Part model, mm, in its own coordinate system. A direction names the side the tool comes from. Round coordinates to 2 decimals unless told otherwise and drop trailing zeros. Write each loop counter-clockwise with the first axis right and the second up, starting at its lowest first coordinate (ties: lowest second). Pieces come first, ordered by that corner, then holes.
1) Which spindle directions (+Z, -Z, +X, -X, +Y, -Y) get a long thin tool onto all of the face, cutting with end or side? Do faces 1 (the flat face through (-51, 254, 22.309)), 2 (the flat face through (-51, 254, -0.691)), 3 (the flat face through (-32, 246, -1.691)). Say none if no direction does.
2) Flat gauge pins, fed straight in: pin 1 (0.8 mm diameter, centred on y = 266, z = 23, fed in from +X); pin 2 (2 mm diameter, centred on x = -52, y = 394, fed in from +Z); pin 3 (24 mm diameter, centred on x = -52.5, y = 151.5, fed in from -Z). Where does each tip first touch, or does it go through?
3) Saw through at A-A on y = 15. Write the cut outline in (x, z).
4) Pull direction Y, two halves, no side cores. Call faces 4 (the flat face through (-51, 500, 11)), 5 (the cylindrical face through (-46.285, 13.085, 10.97)), 6 (the flat face through (-75.904, 246, 11)): +Y half, -Y half, draft (parallel to the pull), parting line (faces both ways), or undercut.
5) Saw through at B-B on y = 301. Write the cut outline in (x, z), and give its area (3 significant figures).
6) Saw through at C-C on x = -41. Write the cut outline in (y, z).
7) Drill centre lines: L1, parallel to Y at x = -48, z = 21.75; L2, parallel to Z at x = -45, y = 388; L3, parallel to X at y = 153, z = 21.5. Where is each one in solid material? Low to high.
```python
from build123d import *

# Parameters (mm, degrees)
BOSS_EXTRUDE1_DEPTH              = 500
SKETCH3_W                        = 30
SKETCH3_H                        = 1
CUT_EXTRUDE1_DEPTH               = 500
M10X1_0_TAPPED_HOLE1_D           = 9
M10X1_0_TAPPED_HOLE1_DEPTH       = 51.26
M10X1_0_TAPPED_HOLE1_CBORE_D     = 10
M10X1_0_TAPPED_HOLE1_CBORE_DEPTH = 45.4
M10X1_0_TAPPED_HOLE1_TIP         = 2.703872786


with BuildPart() as part:
    # Sketch1 → Boss-Extrude1 (new body)
    with BuildSketch(Plane(origin=(0, 0, 0), x_dir=(1, 0, 0), z_dir=(0, 1, 0))):
        with BuildLine():
            Line((-73.903884132, 1.690933219), (-27.903884132, 1.690933219))
            ThreePointArc((-27.903884132, 1.690933219), (-26.48967057, 1.105146782), (-25.903884132, -0.309066781))
            Line((-25.903884132, -0.309066781), (-25.903884132, -21.309066781))
            ThreePointArc((-25.903884132, -21.309066781), (-26.48967057, -22.723280343), (-27.903884132, -23.309066781))
            Line((-27.903884132, -23.309066781), (-73.903884132, -23.309066781))
            ThreePointArc((-73.903884132, -23.309066781), (-75.318097695, -22.723280343), (-75.903884132, -21.309066781))
            Line((-75.903884132, -21.309066781), (-75.903884132, -0.309066781))
            ThreePointArc((-75.903884132, -0.309066781), (-75.318097695, 1.105146782), (-73.903884132, 1.690933219))
        make_face()
    extrude(amount=BOSS_EXTRUDE1_DEPTH)

    # Sketch3 → Cut-Extrude1 (cut)
    with BuildSketch(Plane(origin=(0, 500, 0), x_dir=(1, 0, 0), z_dir=(0, 1, 0))):
        with Locations((-50.903884132, 1.190933219)):
            Rectangle(SKETCH3_W, SKETCH3_H)
        with Locations((-50.903884132, -22.809066781)):
            Rectangle(SKETCH3_W, SKETCH3_H)
    extrude(amount=-CUT_EXTRUDE1_DEPTH, mode=Mode.SUBTRACT)

    # M10x1.0 Tapped Hole1
    with Locations(Plane(origin=(-50.903884132, 485, 22.309066781), x_dir=(1, 0, 0), z_dir=(0, 0, 1))):
        with Locations((0, 0), (0, -470)):
            CounterBoreHole(M10X1_0_TAPPED_HOLE1_D / 2, M10X1_0_TAPPED_HOLE1_CBORE_D / 2, M10X1_0_TAPPED_HOLE1_CBORE_DEPTH, depth=M10X1_0_TAPPED_HOLE1_DEPTH)
            with Locations((0, 0, -(M10X1_0_TAPPED_HOLE1_DEPTH + M10X1_0_TAPPED_HOLE1_TIP / 2))):  # 118° drill point
                Cone(0, M10X1_0_TAPPED_HOLE1_D / 2, M10X1_0_TAPPED_HOLE1_TIP, mode=Mode.SUBTRACT)


solid = part.part
```
Completed:
1. face 1: +Z, +Y, -Y
1. face 2: -Z, +Y, -Y
1. face 3: -Z, +X, -X, +Y, -Y
2. pin 1: stops at x = -26.38
2. pin 2: stops at z = 22.31
2. pin 3: stops at z = -0.69
3. outline: (-75.9, 0.31) arc R2 ccw to (-73.9, -1.69) - (-65.9, -1.69) - (-65.9, -0.69) - (-55.9, -0.69) - (-55.9, 22.31) - (-65.9, 22.31) - (-65.9, 23.31) - (-73.9, 23.31) arc R2 ccw to (-75.9, 21.31) - close; (-45.9, -0.69) - (-35.9, -0.69) - (-35.9, -1.69) - (-27.9, -1.69) arc R2 ccw to (-25.9, 0.31) - (-25.9, 21.31) arc R2 ccw to (-27.9, 23.31) - (-35.9, 23.31) - (-35.9, 22.31) - (-45.9, 22.31) - close
4. face 4: +Y half
4. face 5: undercut
4. face 6: draft
5. outline: (-75.9, 0.31) arc R2 ccw to (-73.9, -1.69) - (-65.9, -1.69) - (-65.9, -0.69) - (-35.9, -0.69) - (-35.9, -1.69) - (-27.9, -1.69) arc R2 ccw to (-25.9, 0.31) - (-25.9, 21.31) arc R2 ccw to (-27.9, 23.31) - (-35.9, 23.31) - (-35.9, 22.31) - (-65.9, 22.31) - (-65.9, 23.31) - (-73.9, 23.31) arc R2 ccw to (-75.9, 21.31) - close
5. area: 1,190 mm2
6. outline: (0, -0.69) - (500, -0.69) - (500, 22.31) - (0, 22.31) - close
7. L1: y = 0 to 10.93, 19.07 to 480.93, 489.07 to 500
7. L2: z = -0.69 to 22.31
7. L3: x = -75.89 to -25.91
